For this review, take the finished solid that the model builds, in its own axes (mm). Face numbers are marked on the shaded views. Round coordinates to 2 decimals unless told otherwise and drop trailing zeros. Write each loop counter-clockwise with the first axis right and the second up, starting at its lowest first coordinate (ties: lowest second). Pieces come first, ordered by that corner, then holes. Notation, with made-up numbers: M 42.5,-24.75 L 98.5,-24.75 A21 cw 98.5,-7.75 Z; hole C 17,-28 d6. An arc over 180 degrees is marked long. Answer in a Markdown table with one row per item.
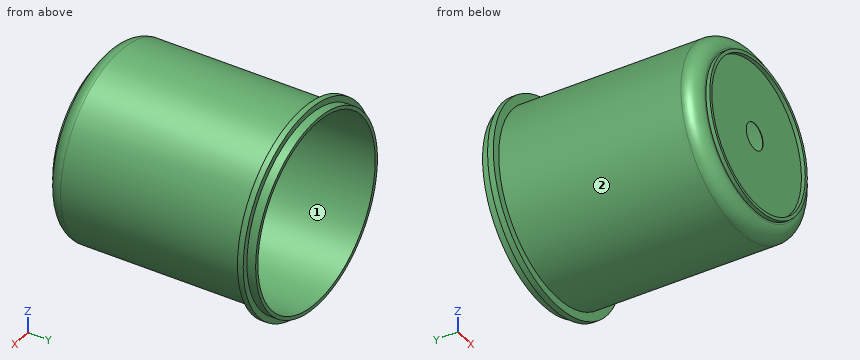
Autodesk Inventor part; units mm, degrees
ref_plane "YZ Plane" through (0, 0, 0) normal (1, 0, 0) x (0, 1, 0)
ref_plane "XZ Plane" through (0, 0, 0) normal (0, 1, 0) x (-1, 0, 0)
ref_plane "XY Plane" through (0, 0, 0) normal (0, 0, 1) x (1, 0, 0)
sketch "Sketch1" plane through (0, 0, 0) normal (0, 0, 1) x (1, 0, 0)
  line L0 (46.8, 0) -> (47.9667, 0)
  line L1 (47.9667, 7.5) -> (47.9667, 101.6997)
  line L2 (47.725, 109.1997) -> (47.525, 109.1997)
  line L3 (47.525, 109.1997) -> (47.525, 7.7)
  line L4 (47.525, 109.1997) -> (49.325, 109.1997)
  line L5 (49.325, 109.1997) -> (49.325, 104.6997)
  line L6 (49.325, 104.6997) -> (52.325, 104.6997)
  line L7 (52.325, 104.6997) -> (52.325, 101.6997)
  line L8 (52.325, 101.6997) -> (49.325, 101.6997)
  line L9 (49.325, 101.6997) -> (47.9667, 101.6997)
  line L10 (0, 0) -> (0, 20.8136)
  line L11 (40.4667, 0) -> (-0.2292, 0)
  line L12 (0, 0) -> (0, 0.2)
  line L13 (0, 0.2) -> (40.025, 0.2)
  arc A0 (40.025, 0.2) -> (47.525, 7.7) centre (40.025, 7.7) ccw
  arc A1 (40.4667, 0) -> (47.9667, 7.5) centre (40.4667, 7.5) ccw
  dimension "d1" = 0.2
  dimension "d2" = 109.2
  dimension "d3" = 1.8
  dimension "d4" = 4.5
  dimension "d5" = 3
  dimension "d6" = 3
  dimension "d7" = 0.2
  dimension "d8" = 90
  dimension "d14" = 7.5
  dimension "d15" = 0.2
revolve "Revolution1" add sketch "Sketch1" angle 360 about axis through (0, 0, 0) along (0, 1, 0)
sketch "Sketch2" plane through (0, 0, 0) normal (0, -1, 0) x (1, 0, 0)
  circle A0 centre (0, 0) radius 6.8
  dimension "d11" = 13.6
extrude "Extrusion1" cut sketch "Sketch2" against normal blind 1
sketch "Sketch3" plane through (0, 0, 0) normal (0, -1, 0) x (1, 0, 0)
  circle A0 centre (0, 0) radius 37.85
  circle A1 centre (0, 0) radius 6.8
  circle A2 centre (0, 0) radius 39.5
  dimension "d16" = 75.7
  dimension "d17" = 79
extrude "Extrusion2" add sketch "Sketch3" along normal blind 2 contours A2
properties part number "ContenedorTest"
Q1. For probe 1 along Z at (x, y) = (1, 78.5); probe 2 along Y at (x, z) = (16, -19); probe 3 along X at (y, z) = (61, 0) (3 decimals), list the stretches that pass through material, from the lowest coordinate up.
Found:
| item | result |
|---|---|
| probe 1 | -47.96 to -47.51, 47.51 to 47.96 |
| probe 2 | 0 to 0.2 |
| probe 3 | -47.967 to -47.525, 47.525 to 47.967 |
Q2. Mouldability with a two-part tool opening along X and no side actions: class the marked faces 1 and 2 as +X half, -X half, draft (parallel to the pull), parting line (faces both ways), or undercut.
Found:
| item | result |
|---|---|
| face 1 | undercut |
| face 2 | parting line |
Q3. Insertion check: P1, Ø1, axis at y = 89.5, z = -21, coming from the -X side; P2, Ø1.5, axis at x = 4, z = 15, coming from the -Y side; P3, Ø3, axis at x = -36, y = 44.5, coming from the +Z side (3 decimals). Each pin has a flat end and moves straight along its axis. Give the tip position at first contact, or say it passes through.
Found:
| item | result |
|---|---|
| P1 | x = -43.37 |
| P2 | y = 0 |
| P3 | z = 33.325 |
Q4. Take a section at C-C (y = 72.5). State the section outline as (x, z) points (3 decimals), then the cut area to 3 significant figures.
Found:
| item | result |
|---|---|
| outline | C 0,0 d95.933; hole C 0,0 d95.05 |
| area | 133 mm² |
